Verification items for this drawing (mm, ordinates from the low corner). A direction names the side the tool comes from. Round coordinates to 2 decimals unless told otherwise and drop trailing zeros. Loops run counter-clockwise (first coordinate to the right, second up) from the corner with the lowest first, then second, coordinate; pieces in that order, holes last. Notation, with made-up numbers: (-23, -33) -> (14, -33) arc R21 cw to (14, 5) -> close; hole circle Ø10 at (-35.5, 85). An arc over 180 degrees is marked (long way). Use a Markdown table: item, result. Add a question column.
Q1. Material ranges on L1, parallel to Y at x = 15, z = 1; L2, parallel to Y at x = 28, z = 4.75; L3, parallel to X at y = 2.5, z = 8.25, recorded low to high.
Q2. Release check for a two-part mould opening along Y. For the marked faces 5, 6, 7 and 8 record: released by +Y, released by -Y, zero draft, split by the parting line, or undercut.
Q3. Sectioned sample at C-C, the plane y = 10.5. Enter the section's corners in (x, z), then the cut area to 3 significant figures.
Q4. Gauge pin test, flat ends, axial feed: P1, Ø1.2, axis at y = 7.5, z = 4, coming from the +X side; P2, Ø1, axis at y = 10, z = 7.5, coming from the -X side. Record the tip position at first contact, or that the pin passes through.
Q5. Set-up check for the marked faces 1, 2, 3 and 4: record each of +Z, -Z, +X, -X, +Y, -Y from which the full face is reachable in a straight line by a thin tool's end or side.
Q6. Sectioned sample at B-B, the plane x = 25.5. Enter the section's corners in (y, z).
Q7. Sectioned sample at A-A, the plane z = 3. Enter the section's corners in (x, y), then the cut area to 3 significant figures.
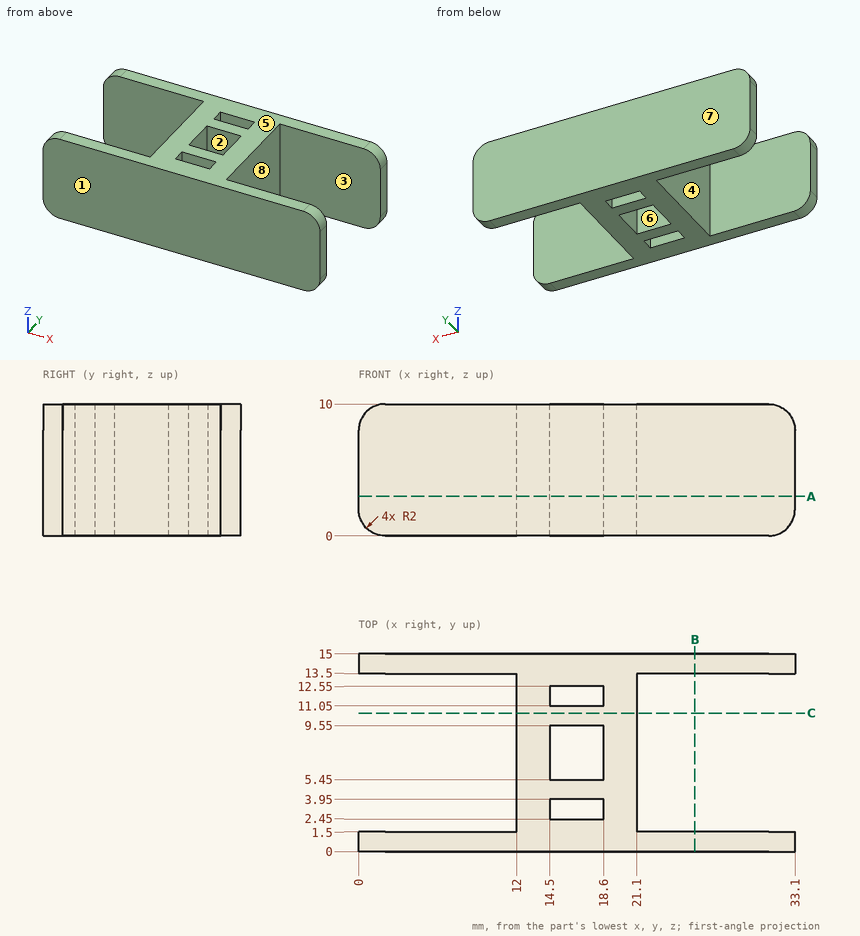
Values:
| question | item | result |
|---|---|---|
| 1 | L1 | 0 to 2.45, 3.95 to 5.45, 9.55 to 11.05, 12.55 to 15 |
| 1 | L2 | 0 to 1.5, 13.5 to 15 |
| 1 | L3 | 12 to 14.5, 18.6 to 21.1 |
| 2 | face 5 | zero draft |
| 2 | face 6 | undercut |
| 2 | face 7 | released by +Y |
| 2 | face 8 | undercut |
| 3 | outline | (12, 0) -> (21.1, 0) -> (21.1, 10) -> (12, 10) -> close |
| 3 | area | 91.0 mm^2 |
| 4 | P1 | x = 21.1 |
| 4 | P2 | x = 12 |
| 5 | face 1 | +Z, -Z, +X, -X, -Y |
| 5 | face 2 | +Z, -Z |
| 5 | face 3 | +Z, -Z, +X |
| 5 | face 4 | +Z, -Z, -X |
| 6 | outline | (0, 0) -> (1.5, 0) -> (1.5, 10) -> (0, 10) -> close; (13.5, 0) -> (15, 0) -> (15, 10) -> (13.5, 10) -> close |
| 7 | outline | (0, 0) -> (33.1, 0) -> (33.1, 1.5) -> (21.1, 1.5) -> (21.1, 13.5) -> (33.1, 13.5) -> (33.1, 15) -> (0, 15) -> (0, 13.5) -> (12, 13.5) -> (12, 1.5) -> (0, 1.5) -> close; hole (14.5, 2.45) -> (18.6, 2.45) -> (18.6, 3.95) -> (14.5, 3.95) -> close; hole (14.5, 5.45) -> (18.6, 5.45) -> (18.6, 9.55) -> (14.5, 9.55) -> close; hole (14.5, 11.05) -> (18.6, 11.05) -> (18.6, 12.55) -> (14.5, 12.55) -> close |
| 7 | area | 179 mm^2 |
